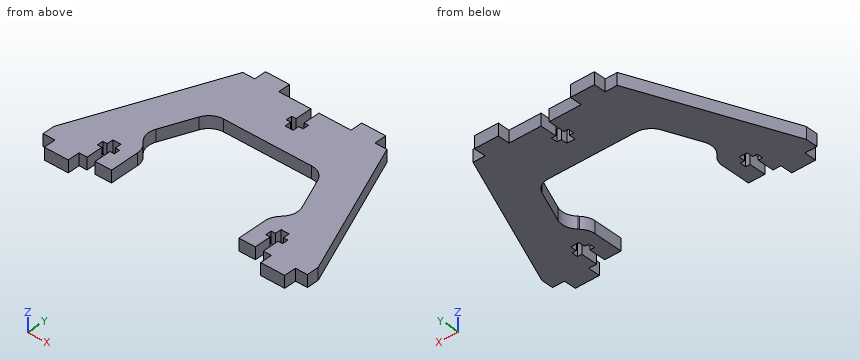
from build123d import *

# Parameters (mm, degrees)
SKETCH1_W               = 139.7
SKETCH1_H               = 82.55
BOSS_EXTRUDE1_DEPTH     = 6.35
SKETCH2_W               = 12.7
SKETCH2_H               = 6.35
BOSS_EXTRUDE2_DEPTH     = 6.35
CUT_EXTRUDE1_DEPTH      = 6.35
CUT_EXTRUDE8_DEPTH      = 6.35
CUT_EXTRUDE2_DEPTH      = 6.35
CUT_EXTRUDE9_DEPTH      = 85.77904001
CUT_EXTRUDE9_DEPTH_BACK = 85.77904001
FILLET1_R               = 8.89


with BuildPart() as part:
    # Sketch1 → Boss-Extrude1 (new body)
    with BuildSketch(Plane.XY):
        Rectangle(SKETCH1_W, SKETCH1_H)
    extrude(amount=BOSS_EXTRUDE1_DEPTH)

    # Sketch2 → Boss-Extrude2 (add)
    with BuildSketch(Plane(origin=(0, 0, 0), x_dir=(-1, 0, 0), z_dir=(0, 0, -1))):
        with Locations((-57.15, -44.45)):
            Rectangle(SKETCH2_W, SKETCH2_H)
        with Locations((-25.4, 44.45)):
            Rectangle(SKETCH2_W, SKETCH2_H)
    boss_extrude2 = extrude(amount=-BOSS_EXTRUDE2_DEPTH)

    # Sketch3 → Cut-Extrude1 (cut)
    with BuildSketch(Plane(origin=(0, 0, 0), x_dir=(-1, 0, 0), z_dir=(0, 0, -1))):
        Polygon((-46.5836, -41.275), (-46.5836, -32.512), (-48.895, -32.512), (-48.895, -29.337), (-46.5836, -29.337), (-46.5836, -26.035), (-42.3164, -26.035), (-42.3164, -29.337), (-40.005, -29.337), (-40.005, -32.512), (-42.3164, -32.512), (-42.3164, -41.275), align=None)
    cut_extrude1 = extrude(amount=-CUT_EXTRUDE1_DEPTH, mode=Mode.SUBTRACT)

    # Sketch7 → Cut-Extrude8 (cut)
    with BuildSketch(Plane(origin=(0, 0, 0), x_dir=(-1, 0, 0), z_dir=(0, 0, -1))):
        Polygon((-38.1, 41.275), (-69.85, -34.925), (-69.85, 41.275), align=None)
    cut_extrude8 = extrude(amount=-CUT_EXTRUDE8_DEPTH, mode=Mode.SUBTRACT)

    # Mirror2: Boss-Extrude2, Cut-Extrude8 across plane
    add(boss_extrude2.mirror(Plane(origin=(0, 0, 0), x_dir=(0, 0, 1), z_dir=(1, 0, 0))))
    add(cut_extrude8.mirror(Plane(origin=(0, 0, 0), x_dir=(0, 0, 1), z_dir=(1, 0, 0))), mode=Mode.SUBTRACT)

    # Mirror4: Cut-Extrude1 across plane
    add(cut_extrude1.mirror(Plane(origin=(0, 0, 0), x_dir=(0, 0, 1), z_dir=(1, 0, 0))), mode=Mode.SUBTRACT)

    # Sketch4 → Cut-Extrude2 (cut)
    with BuildSketch(Plane(origin=(0, 0, 0), x_dir=(-1, 0, 0), z_dir=(0, 0, -1))):
        Polygon((2.1336, 41.275), (-2.1336, 41.275), (-2.1336, 32.512), (-4.445, 32.512), (-4.445, 29.337), (-2.1336, 29.337), (-2.1336, 26.035), (2.1336, 26.035), (2.1336, 29.337), (4.445, 29.337), (4.445, 32.512), (2.1336, 32.512), align=None)
    extrude(amount=-CUT_EXTRUDE2_DEPTH, mode=Mode.SUBTRACT)

    # Sketch8 → Cut-Extrude9 (cut, two sides: drawn at the far end of the back side and taken through both)
    with BuildSketch(Plane.XY.offset(6.35).offset(-CUT_EXTRUDE9_DEPTH_BACK)):
        Polygon((-33.655, -22.225), (-40.901470588, -14.978529412), (-29.104166667, 13.335), (29.104166667, 13.335), (40.901470588, -14.978529412), (33.655, -22.225), (33.655, -41.275), (-33.655, -41.275), align=None)
    extrude(amount=CUT_EXTRUDE9_DEPTH + CUT_EXTRUDE9_DEPTH_BACK, mode=Mode.SUBTRACT)

    # Fillet1
    fillet1_edges = [part.edges().sort_by_distance(p)[0] for p in [
        (-33.655, -22.225, 3.175),
        (-40.901470588, -14.978529412, 3.175),
        (-29.104166667, 13.335, 3.175),
        (29.104166667, 13.335, 3.175),
        (40.901470588, -14.978529412, 3.175),
        (33.655, -22.225, 3.175),
    ]]
    fillet(fillet1_edges, radius=FILLET1_R)


solid = part.part
Build history of the part. All positions in model axes, mm. Round coordinates to 2 decimals unless told otherwise and drop trailing zeros. Write each loop counter-clockwise with the first axis right and the second up, starting at its lowest first coordinate (ties: lowest second). Pieces come first, ordered by that corner, then holes. Notation, with made-up numbers: (-9, 20.25) -> (22, 20.25) arc R35 ccw to (22, 54.25) -> close; hole circle Ø1 at (8, 4.5). An arc over 180 degrees is marked (long way). Write item = value, one per line.
(1) Probe L1, parallel to X at y = -38, z = 1.5 (3 decimals); L2, parallel to X at y = -34, z = 2.75 (3 decimals); L3, parallel to X at y = 3.5, z = 5.5. List the from-to ranges inside material, lowest first.
Answer:
L1 = -69.85 to -46.584, -42.316 to -33.655, 33.655 to 42.316, 46.584 to 69.85
L2 = -69.465 to -46.584, -42.316 to -33.655, 33.655 to 42.316, 46.584 to 69.465
L3 = -53.84 to -33.2, 33.2 to 53.84
(2) Flat gauge pins, fed straight in: pin 1 (3 mm diameter, centred on y = 44.5, z = 4.5, fed in from +X); pin 2 (3.5 mm diameter, centred on y = 28.5, z = 4, fed in from -X); pin 3 (2.5 mm diameter, centred on x = 41.5, z = 2.5, fed in from -Y) (3 decimals). Where does each tip first touch, or does it go through?
Answer:
pin_1 = 31.75
pin_2 = -44.15
pin_3 = -41.275
(3) Band-saw the part on A-A (y = -39). Give the cut face in (x, z) (3 decimals).
Answer:
outline = (-69.85, 0) -> (-46.584, 0) -> (-46.584, 6.35) -> (-69.85, 6.35) -> close; (-42.316, 0) -> (-33.655, 0) -> (-33.655, 6.35) -> (-42.316, 6.35) -> close; (33.655, 0) -> (42.316, 0) -> (42.316, 6.35) -> (33.655, 6.35) -> close; (46.584, 0) -> (69.85, 0) -> (69.85, 6.35) -> (46.584, 6.35) -> close
(4) Band-saw the part on C-C (x = 13). Give the cut face in (y, z) (3 decimals), then the cut area to 3 significant figures.
Answer:
outline = (13.335, 0) -> (41.275, 0) -> (41.275, 6.35) -> (13.335, 6.35) -> close
area = 177 mm2
(5) Band-saw the part on B-B (y = -22). Give the cut face in (x, z), then the cut area to 3 significant figures.
Answer:
outline = (-64.46, 0) -> (-34.56, 0) -> (-34.56, 6.35) -> (-64.46, 6.35) -> close; (34.56, 0) -> (64.46, 0) -> (64.46, 6.35) -> (34.56, 6.35) -> close
area = 380 mm2
(6) Band-saw the part on D-D (y = 20.5). Give the cut face in (x, z), then the cut area to 3 significant figures.
Answer:
outline = (-46.76, 0) -> (46.76, 0) -> (46.76, 6.35) -> (-46.76, 6.35) -> close
area = 594 mm2
